For this review, take the finished solid that the model builds, in its own axes (mm). A direction names the side the tool comes from. Coordinates: 2 decimals unless noted, no trailing zeros. Loops run counter-clockwise (first coordinate to the right, second up) from the corner with the lowest first, then second, coordinate; pieces in that order, holes last. Notation, with made-up numbers: (81.5, 34.25) - (89.5, 34.25) arc R31 ccw to (89.5, 61.25) - close; hole circle Ø1 at (64, 75.25). An arc over 180 degrees is marked (long way). One line per item, written item: value. Start each with the question number.
1. Take a section at C-C, the plane x = 18.5. State the section outline as (y, z) points, and give its area (3 significant figures).
2. For faces 5 (the face through (2.285, 3.584, 4.746)), 6 (the face through (-4.03, -16.98, 0.99)), 7 (the face through (17, 5, 1)), 8 (the face through (0, -1, 3)), 9 (the face through (-12.7, 12, 1)), list the 3-axis set-ups (+Z, -Z, +X, -X, +Y, -Y) from which the entire face can be reached by the end or side of a thin tool; tool diameter is ignored.
3. Insertion check: pin 1 (0.6 mm diameter, centred on x = 16.5, z = 1.5, fed in from +Y); pin 2 (3 mm diameter, centred on x = 16.5, y = -4, fed in from +Z); pin 3 (1.2 mm diameter, centred on x = 0, y = 0, fed in from -Z); pin 4 (24 mm diameter, centred on x = 5.5, y = -12.5, fed in from +Z). Each pin has a flat end and moves straight along its axis. Give the tip position at first contact, or say it passes through.
4. Take a section at D-D, the plane y = 18. State the section outline as (x, z) points.
5. To check wall thickness, follow line 1 (X direction, y = 0, z = 1.35); line 2 (Z direction, x = -6.5, y = -3.5); line 3 (Y direction, x = 3, z = 1.1). State the ranges of each line that lie inside material, in increasing order. Write a range as from..to.
6. The part is to be moulded in two halves that separate along Y. For faces 1 (the face through (-7.32, -0.07, 1.01)), 2 (the face through (17, -5, 1)), 3 (the face through (-4.03, 16.98, 0.99)), 4 (the face through (-17.35, 22.89, 1.01)), say which applies: released by +Y, released by -Y, zero draft, split by the parting line, or undercut.
7. Take a section at B-B, the plane x = -12.5. State the section outline as (y, z) points.
```python
from build123d import *

# Parameters (mm, degrees)
CYLINDER_R        = 1
CYLINDER_DEPTH    = 10
CYLINDER001_R     = 4.25
CYLINDER001_DEPTH = 6
BOX_W             = 30
BOX_H             = 10
BOX_DEPTH         = 2
ARRAY_COUNT       = 3
FILLET_1_R        = 10
FILLET_2_R        = 4.99
FILLET001_1_R     = 2.5
FILLET001_2_R     = 1


with BuildPart() as hueco_eje_central:
    # Cylinder → Cylinder (new body)
    with BuildSketch(Plane.XY.offset(-2)):
        Circle(CYLINDER_R)
    extrude(amount=CYLINDER_DEPTH)


with BuildPart() as cilindro_base_soporte:
    # Cylinder001 → Cylinder001 (new body)
    with BuildSketch(Plane.XY):
        Circle(CYLINDER001_R)
    extrude(amount=CYLINDER001_DEPTH)


with BuildPart() as obj1:
    # Box → Box (new body)
    with BuildSketch(Plane(origin=(0, -5, 0), x_dir=(1, 0, 0), z_dir=(0, 0, 1))):
        with Locations((15, 5)):
            Rectangle(BOX_W, BOX_H)
    extrude(amount=BOX_DEPTH)

    # Array: obj1 ×3 about axis
    array_axis = Axis((0, 0, 0), (0, 0, 1))


with BuildPart() as obj1_1:
    add(obj1.part)
    for i in range(1, ARRAY_COUNT):
        add(obj1.part.rotate(array_axis, i * 360 / ARRAY_COUNT))

    # Fillet 1
    fillet_1_edges = [obj1_1.edges().sort_by_distance(p)[0] for p in [
        (2.886751, -5, 1),
        (2.886751, 5, 1),
        (-5.773503, 0, 1),
    ]]
    fillet(fillet_1_edges, radius=FILLET_1_R)

    # Fillet 2
    fillet_2_edges = [obj1_1.edges().sort_by_distance(p)[0] for p in [
        (30, -5, 1),
        (30, 5, 1),
        (-10.669873, -28.480762, 1),
        (-10.669873, 28.480762, 1),
        (-19.330127, -23.480762, 1),
        (-19.330127, 23.480762, 1),
    ]]
    fillet(fillet_2_edges, radius=FILLET_2_R)

    # Fusion001: union Cilindro base soporte
    add(cilindro_base_soporte.part)

    # Fillet001 1
    fillet001_1_edges = [obj1_1.edges().sort_by_distance(p)[0] for p in [
        (-4.25, 0, 2),
    ]]
    fillet(fillet001_1_edges, radius=FILLET001_1_R)

    # Fillet001 2
    fillet001_2_edges = [obj1_1.edges().sort_by_distance(p)[0] for p in [
        (-4.25, 0, 6),
    ]]
    fillet(fillet001_2_edges, radius=FILLET001_2_R)

    # Cut: cut hueco eje central
    add(hueco_eje_central.part, mode=Mode.SUBTRACT)


solid = obj1_1.part
```
Solutions:
1. outline: (-5, 0) - (5, 0) - (5, 2) - (-5, 2) - close
1. area: 20.0 mm2
2. face 5: +Z
2. face 6: +Z, -Z, +X, -Y
2. face 7: +Z, -Z, +X, +Y
2. face 8: +Z, -Z
2. face 9: +Z, -Z, -X
3. pin 1: y = 5
3. pin 2: z = 2
3. pin 3: through
3. pin 4: z = 6
4. outline: (-16.17, 0) - (-4.62, 0) - (-4.62, 2) - (-16.17, 2) - close
5. line 1: -7.32..-1, 1..30
5. line 2: 0..2
5. line 3: -6.76..6.76
6. face 1: undercut
6. face 2: released by -Y
6. face 3: released by +Y
6. face 4: undercut
7. outline: (-26.65, 0) - (-11.65, 0) - (-11.65, 2) - (-26.65, 2) - close; (11.65, 0) - (26.65, 0) - (26.65, 2) - (11.65, 2) - close
